from build123d import *

# Parameters (mm, degrees)
SKETCH1_W           = 29
SKETCH1_H           = 40
BOSS_EXTRUDE1_DEPTH = 10
SKETCH2_R           = 7.6
CUT_EXTRUDE1_DEPTH  = 40
SKETCH3_R           = 1.5
CUT_EXTRUDE2_DEPTH  = 10


with BuildPart() as part:
    # Sketch1 → Boss-Extrude1 (new body)
    with BuildSketch(Plane(origin=(0, 0, 0), x_dir=(0, 1, 0), z_dir=(0, 0, 1))):
        with Locations((14.5, -20)):
            Rectangle(SKETCH1_W, SKETCH1_H)
    extrude(amount=BOSS_EXTRUDE1_DEPTH)

    # Sketch2 → Cut-Extrude1 (cut)
    with BuildSketch(Plane.YZ.offset(40)):
        with Locations((14.5, 10)):
            Circle(SKETCH2_R)
    extrude(amount=-CUT_EXTRUDE1_DEPTH, mode=Mode.SUBTRACT)

    # Sketch3 → Cut-Extrude2 (cut)
    with BuildSketch(Plane.XY.offset(10)):
        with Locations((6.45, 25.55)):
            Circle(SKETCH3_R)
        with Locations((33.55, 25.55)):
            Circle(SKETCH3_R)
        with Locations((33.55, 3.45)):
            Circle(SKETCH3_R)
        with Locations((6.45, 3.45)):
            Circle(SKETCH3_R)
    extrude(amount=-CUT_EXTRUDE2_DEPTH, mode=Mode.SUBTRACT)


solid = part.part
Source: CAD feature listing. Evaluate the final solid. Frame: model axes, mm. Coordinates: 2 decimals unless noted, no trailing zeros. Order: outer loops, then holes, each group sorted by start corner. A loop starts at its lowest first (then second) coordinate and runs counter-clockwise, first axis right, second up.
Item 1: Pull-direction query (X, two-part tool) for faces 1 (the face through (0, 14, 2)), 2 (the face through (20, 3, 10)), 3 (the face through (6.125, 24.086, 5.07)); classes: pulls with the +X half, pulls with the -X half, needs draft (parallel to the pull), parting line crosses it, or undercut.
Output values:
face 1: pulls with the -X half
face 2: needs draft
face 3: undercut
Item 2: Material intervals for line 1 (Y direction, x = 6.45, z = 4.25); line 2 (Y direction, x = 6.45, z = 6.75); line 3 (X direction, y = 24.5, z = 8), sorted ascending.
Output values:
line 1: y = 0 to 1.95, 4.95 to 9.53, 19.47 to 24.05, 27.05 to 29
line 2: y = 0 to 1.95, 4.95 to 7.63, 21.37 to 24.05, 27.05 to 29
line 3: x = 0 to 5.38, 7.52 to 32.48, 34.62 to 40
Item 3: Cut plane D-D (z = 0.5). Return loops of the section in (x, y), plus the area to 3 significant figures.
Output values:
outline: (0, 0) - (40, 0) - (40, 29) - (0, 29) - close; hole circle Ø3 at (6.45, 3.45); hole circle Ø3 at (6.45, 25.55); hole circle Ø3 at (33.55, 3.45); hole circle Ø3 at (33.55, 25.55)
area: 1,130 mm2
Item 4: Cut plane C-C (y = 3.45). Return loops of the section in (x, z), plus the area to 3 significant figures.
Output values:
outline: (0, 0) - (4.95, 0) - (4.95, 10) - (0, 10) - close; (7.95, 0) - (32.05, 0) - (32.05, 10) - (7.95, 10) - close; (35.05, 0) - (40, 0) - (40, 10) - (35.05, 10) - close
area: 340 mm2
Item 5: First-contact query: P1, Ø2.5, axis at x = 6.45, y = 3.45, coming from the +Z side; P2, Ø4, axis at x = 15.5, y = 16, coming from the +Z side. Flat tips, straight axial feed; report the tip coordinate or a pass-through.
Output values:
P1: passes through
P2: stops at z = 3.25
Item 6: Cut plane B-B (z = 3). Return loops of the section in (x, y).
Output values:
outline: (0, 0) - (40, 0) - (40, 11.54) - (0, 11.54) - close; (0, 17.46) - (40, 17.46) - (40, 29) - (0, 29) - close; hole circle Ø3 at (6.45, 3.45); hole circle Ø3 at (6.45, 25.55); hole circle Ø3 at (33.55, 3.45); hole circle Ø3 at (33.55, 25.55)
Item 7: Cut plane A-A (x = 33.55). Return loops of the section in (y, z).
Output values:
outline: (0, 0) - (1.95, 0) - (1.95, 10) - (0, 10) - close; (4.95, 0) - (24.05, 0) - (24.05, 10) - (22.1, 10) arc R7.6 cw to (6.9, 10) - (4.95, 10) - close; (27.05, 0) - (29, 0) - (29, 10) - (27.05, 10) - close
